Could you check a few things on this model? Use its own coordinates, in mm. A direction names the side the tool comes from. Coordinates: 2 decimals unless noted, no trailing zeros. Write each loop counter-clockwise with the first axis right and the second up, starting at its lowest first coordinate (ties: lowest second). Pieces come first, ordered by that corner, then holes.
```python
from build123d import *

# Parameters (mm, degrees)
ESQUISSE1_R                  = 1.050000000000002
ESQUISSE1_R_2                = 0.5500000000000002
BOSS_EXTRU_1_DEPTH           = 5.588
BOSS_EXTRU_2_START           = 10.16
BOSS_EXTRU_2_DEPTH           = 10.16
ESQUISSE3_W                  = 7.349999
ESQUISSE3_H                  = 12.302264747859223
ENL_V_MAT_EXTRU_1_DEPTH      = 5.715
CONG_1_R                     = 10.16
CONG_2_R                     = 5.08
ENL_V_MAT_EXTRU_2_DEPTH      = 58.09584154270072
ENL_V_MAT_EXTRU_2_DEPTH_BACK = 58.09584154270072
ESQUISSE4_R                  = 1.050000000000002
CONG_3_R                     = 1.5


with BuildPart() as part:
    # Esquisse1 → Boss.-Extru.1 (new body)
    with BuildSketch(Plane(origin=(0, 0, 0), x_dir=(0, 0, -1), z_dir=(1, 0, 0))):
        with BuildLine():
            ThreePointArc((-34.925000000000004, 0), (-30.245937227171517, 17.462500000000013), (-17.4625, 30.245937227171524))
            ThreePointArc((-17.4625, 30.245937227171524), (-16.300369342984403, 34.583067884187116), (-20.637499999999996, 35.745198541202704))
            ThreePointArc((-20.637499999999996, 35.745198541202704), (-35.7451985412027, 20.637500000000014), (-41.275, 0))
            ThreePointArc((-41.275, 0), (-38.1, -3.174999999999997), (-34.925000000000004, 0))
        make_face()
        with Locations((-38.1, 0)):
            Circle(ESQUISSE1_R, mode=Mode.SUBTRACT)
        with Locations((-19.049999999999997, 32.99556788418712)):
            Circle(ESQUISSE1_R_2, mode=Mode.SUBTRACT)
    extrude(amount=BOSS_EXTRU_1_DEPTH)

    # Esquisse2 → Boss.-Extru.2 (add)
    with BuildSketch(Plane.ZY.offset(BOSS_EXTRU_2_START)):
        with BuildLine():
            Line((40.13567832123378, 9.630833333333326), (33.96095857950552, 8.14916666666666))
            ThreePointArc((33.96095857950552, 8.14916666666666), (34.68315227447781, 4.10299565017866), (34.925000000000004, 0))
            ThreePointArc((34.925000000000004, 0), (38.1, -3.174999999999997), (41.275, 0))
            ThreePointArc((41.275, 0), (40.9891799607465, 4.848994859302054), (40.13567832123378, 9.630833333333326))
        make_face()
    extrude(amount=-BOSS_EXTRU_2_DEPTH)

    # Esquisse3 → Enlèv. mat.-Extru.1 (cut, symmetric)
    with BuildSketch(Plane(origin=(0, 0, 0), x_dir=(1, 0, 0), z_dir=(0, 1, 0))):
        with Locations((-3.2647804999577055, -37.13499681447274)):
            Rectangle(ESQUISSE3_W, ESQUISSE3_H)
    extrude(amount=ENL_V_MAT_EXTRU_1_DEPTH, both=True, mode=Mode.SUBTRACT)

    # Congé1
    cong_1_edges = [part.edges().sort_by_distance(p)[0] for p in [
        (0, 8.889999999999993, 37.04831845036965),
    ]]
    fillet(cong_1_edges, radius=CONG_1_R - 0.0001)  # a hair under: the kernel refuses the full size

    # Congé2
    cong_2_edges = [part.edges().sort_by_distance(p)[0] for p in [
        (-10.16, 8.889999999999993, 37.04831845036965),
    ]]
    fillet(cong_2_edges, radius=CONG_2_R)

    # Esquisse4 → Enlèv. mat.-Extru.2 (cut, two sides: drawn at the far end of the back side and taken through both)
    with BuildSketch(Plane(origin=(5.588, 0, 0), x_dir=(0, 0, -1), z_dir=(1, 0, 0)).offset(-ENL_V_MAT_EXTRU_2_DEPTH_BACK)):
        with Locations(Location((-38.10000264654745, -3.51466647443e-06, 0), (0, 0, 0.000191786))):
            Circle(ESQUISSE4_R)
    extrude(amount=ENL_V_MAT_EXTRU_2_DEPTH + ENL_V_MAT_EXTRU_2_DEPTH_BACK, mode=Mode.SUBTRACT)

    # Congé3
    cong_3_edges = [part.edges().sort_by_distance(p)[0] for p in [
        (-3.2647804999577055, 5.715, 40.87743142615494),
        (-3.2647804999577055, 5.715, 34.45423631427637),
    ]]
    fillet(cong_3_edges, radius=CONG_3_R)


solid = part.part
```
1. I want a section at B-B on x = 4.75. Give the number of separate pieces and of enclosed holes in the cut face, plus the area to 3 significant figures.
Verdict:
separate pieces: 1
enclosed holes: 2
area: 281 mm2
2. I want a section at C-C on x = -1.5. Please give me the cut outline in (y, z) (3 decimals).
Verdict:
outline: (5.715, 35.703) arc R1.5 ccw to (6.918, 34.233) arc R34.925 cw to (12.783, 32.501) - (14.277, 38.727) arc R41.275 ccw to (7.487, 40.59) arc R1.5 ccw to (5.715, 39.115) - close
3. I want a section at A-A on z = 19.05. Please give me the cut outline in (x, y), plus the area to 3 significant figures.
Verdict:
outline: (0, 29.27) - (5.59, 29.27) - (5.59, 32.45) - (0, 32.45) - close; (0, 33.55) - (5.59, 33.55) - (5.59, 36.17) - (0, 36.17) - close
area: 32.4 mm2
4. On a 3-axis mill with a long thin cutter (end or side, diameter ignored), from which of +Z, -Z, +X, -X, +Y, -Y can I reach the whole of each face in a straight line? I mean faces 4 (the face through (-8.572, -3.174, 38.03)), 5 (the face through (-3, 5.715, 37)), 6 (the face through (-3.3, 6.1, 34.7)). Say none if no direction works.
Verdict:
face 4: +X, -X, -Y
face 5: +Z, -Z, -Y
face 6: -Z, -Y
5. Please list where these lines run through material, in increasing order: line 1 along X through (y, z) = (25.5, 28); line 2 along Y through (x, z) = (1.65, 19.05); line 3 along Z through (x, y) = (2.5, 21).
Verdict:
line 1: x = 0 to 5.59
line 2: y = 29.27 to 32.45, 33.55 to 36.17
line 3: z = 27.91 to 35.53
6. For pin 1 (12 mm diameter, centred on y = 27.5, z = 24, fed in from -X); pin 2 (1 mm diameter, centred on x = 2, z = 36, fed in from -Y); pin 3 (4 mm diameter, centred on x = -0.5, y = 6, fed in from -Z), each with a flat end and sliding along its axis, tell me the tip position at first contact or that it passes through.
Verdict:
pin 1: stops at x = 0
pin 2: stops at y = -2.74
pin 3: stops at z = 34
7. If we mould it in two halves opening along Y, with no side actions, what happens to faces 1 (the face through (-8.57, 0.32, 37.1)), 2 (the face through (5.588, 20, 31)), 3 (the face through (1.1, 16.07, 38.02))? For each: pulls with the +Y half, pulls with the -Y half, needs draft (parallel to the pull), parting line crosses it, or undercut.
Verdict:
face 1: undercut
face 2: needs draft
face 3: pulls with the +Y half
